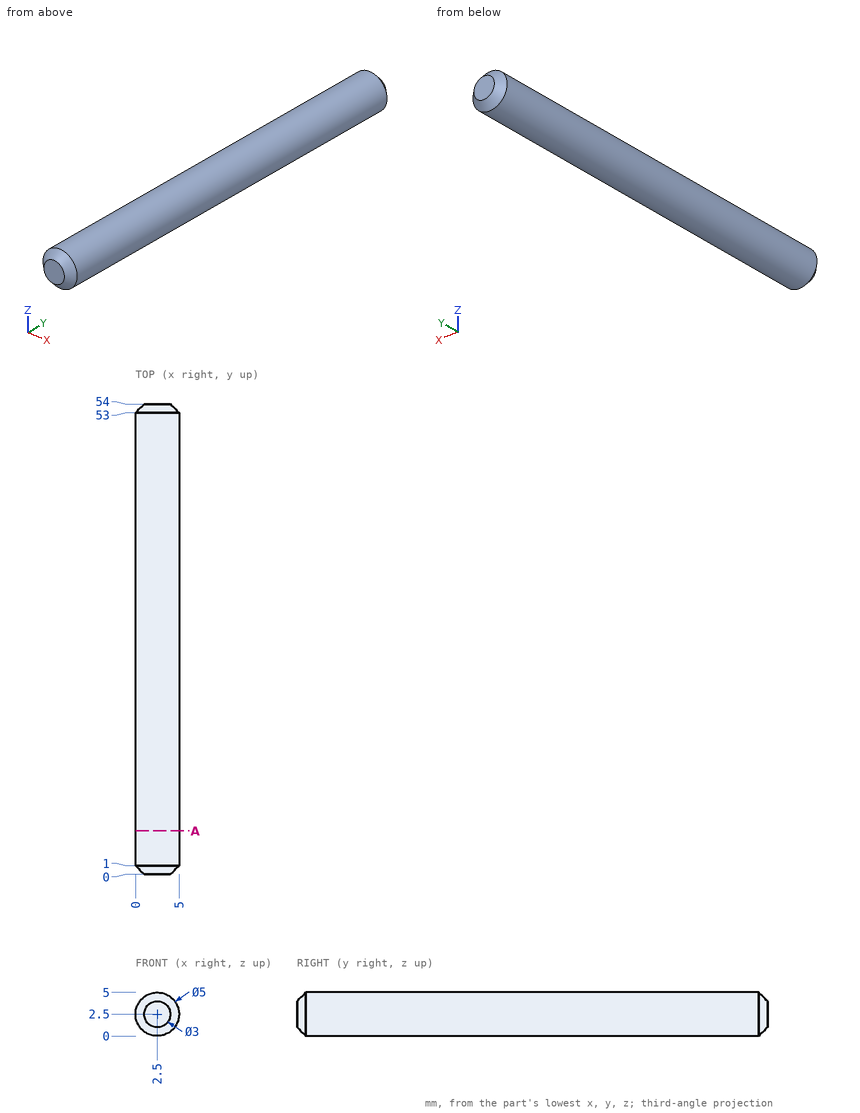
Part print with two shaded views. Sizes in mm from the minimum x, y, z corner. Coordinates: 2 decimals unless noted, no trailing zeros. Order: outer loops, then holes, each group sorted by start corner. A loop starts at its lowest first (then second) coordinate and runs counter-clockwise, first axis right, second up. Notation, with made-up numbers: M 77.5,35 L 129.5,35 A11 ccw 129.5,56 Z; hole C -32.75,65.25 d6. An arc over 180 degrees is marked long. Use a Markdown table: item, result.
(1) Flat gauge pins, fed straight in: pin 1 (1 mm diameter, centred on x = 4, y = 25, fed in from +Z); pin 2 (1 mm diameter, centred on x = 1.5, y = 38.5, fed in from -Z). Where does each tip first touch, or does it go through?
A:
| item | result |
|---|---|
| pin 1 | stops at z = 4.79 |
| pin 2 | stops at z = 0.05 |
(2) Probe L1, parallel to X at y = 47, z = 0.5; L2, parallel to X at y = 22, z = 2.7; L3, parallel to Y at x = 1.7, z = 3.95. List the from-to ranges inside material, lowest first.
A:
| item | result |
|---|---|
| L1 | x = 1 to 4 |
| L2 | x = 0.01 to 4.99 |
| L3 | y = 0.16 to 53.84 |
(3) Cut at A-A on y = 5. Write the cut outline in (x, z).
A:
| item | result |
|---|---|
| outline | C 2.5,2.5 d5 |
